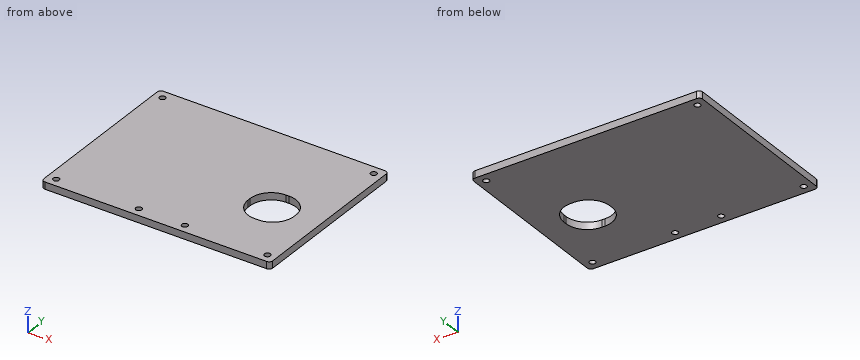
```python
from build123d import *

# Parameters (mm, degrees)
BOSS_EXTRUDE1_DEPTH  = 4
M3_CLEARANCE_HOLE1_D = 3.4
SKETCH4_W            = 25.893128439
SKETCH4_H            = 25.556513708
CUT_EXTRUDE1_DEPTH   = 8
FILLET1_R            = 12


with BuildPart() as part:
    # Sketch1 → Boss-Extrude1 (new body)
    with BuildSketch(Plane.XY):
        with BuildLine():
            Line((-118.577385132, 31.787530767), (6.585636131, 31.787530767))
            ThreePointArc((6.585636131, 31.787530767), (7.999849693, 32.373317205), (8.585636131, 33.787530767))
            Line((8.585636131, 33.787530767), (8.585636131, 127.40770823))
            ThreePointArc((8.585636131, 127.40770823), (7.999849693, 128.821921793), (6.585636131, 129.40770823))
            Line((6.585636131, 129.40770823), (-118.577385132, 129.40770823))
            ThreePointArc((-118.577385132, 129.40770823), (-119.991598694, 128.821921793), (-120.577385132, 127.40770823))
            Line((-120.577385132, 127.40770823), (-120.577385132, 33.787530767))
            ThreePointArc((-120.577385132, 33.787530767), (-119.991598694, 32.373317205), (-118.577385132, 31.787530767))
        make_face()
    extrude(amount=BOSS_EXTRUDE1_DEPTH)

    # M3 Clearance Hole1 (through all)
    with Locations(Plane.XY.offset(4)):
        with Locations((-115.577385132, 124.40770823), (3.585636131, 124.40770823), (-115.577385132, 36.787530767), (-68.995874501, 36.787530767), (-43.015256757, 36.787530767), (3.585636131, 36.787530767)):
            Hole(M3_CLEARANCE_HOLE1_D / 2)

    # Sketch4 → Cut-Extrude1 (cut)
    with BuildSketch(Plane.XY.offset(4)):
        with Locations((-18.472781595, 72.793183927)):
            Rectangle(SKETCH4_W, SKETCH4_H)
    extrude(amount=-CUT_EXTRUDE1_DEPTH, mode=Mode.SUBTRACT)

    # Fillet1
    fillet1_edges = [part.edges().sort_by_distance(p)[0] for p in [
        (-5.526217375, 85.571440781, 2),
        (-5.526217375, 60.014927073, 2),
        (-31.419345814, 60.014927073, 2),
        (-31.419345814, 85.571440781, 2),
    ]]
    fillet(fillet1_edges, radius=FILLET1_R)


solid = part.part
```
Source: CAD feature listing. Evaluate the final solid. Frame: model axes, mm. Coordinates: 2 decimals unless noted, no trailing zeros. Loops run counter-clockwise (first coordinate to the right, second up) from the corner with the lowest first, then second, coordinate; pieces in that order, holes last. Notation, with made-up numbers: M 66.5,-3 L 89.5,-3 A23 cw 89.5,15 Z; hole C 86,68 d10. An arc over 180 degrees is marked long. Use a Markdown table: item, result. Add a question column.
Q1. Section query C-C, the plane y = 62.5. Return loops of the section in (x, z).
Q2. Material intervals for L1, parallel to Y at x = -12.5, z = 1.2; L2, parallel to X at y = 61.5, z = 2.6; L3, parallel to Y at x = -11, z = 3.4, sorted ascending.
Q3. Section query B-B, the plane z = 2. Return loops of the section in (x, y).
Q4. Section query A-A, the plane y = 83. Return loops of the section in (x, z).
Result:
| question | item | result |
|---|---|---|
| 1 | outline | M -120.58,0 L -26.73,0 L -26.73,4 L -120.58,4 Z; M -10.21,0 L 8.59,0 L 8.59,4 L -10.21,4 Z |
| 2 | L1 | y = 31.79 to 61.12, 84.47 to 129.41 |
| 2 | L2 | x = -120.58 to -25.2, -11.74 to 8.59 |
| 2 | L3 | y = 31.79 to 61.94, 83.64 to 129.41 |
| 3 | outline | M -120.58,33.79 A2 ccw -118.58,31.79 L 6.59,31.79 A2 ccw 8.59,33.79 L 8.59,127.41 A2 ccw 6.59,129.41 L -118.58,129.41 A2 ccw -120.58,127.41 Z; hole C -115.58,36.79 d3.4; hole C -115.58,124.41 d3.4; hole C -69,36.79 d3.4; hole C -43.02,36.79 d3.4; hole M -31.42,72.01 A12 ccw -19.42,60.01 L -17.53,60.01 A12 ccw -5.53,72.01 L -5.53,73.57 A12 ccw -17.53,85.57 L -19.42,85.57 A12 ccw -31.42,73.57 Z; hole C 3.59,36.79 d3.4; hole C 3.59,124.41 d3.4 |
| 4 | outline | M -120.58,0 L -26.84,0 L -26.84,4 L -120.58,4 Z; M -10.1,0 L 8.59,0 L 8.59,4 L -10.1,4 Z |
